from build123d import *

# Parameters (mm, degrees)
EXTRUDE_1_DEPTH     = 5
SKETCH_4_W          = 22
SKETCH_4_H          = 15
SKETCH_4_W_2        = 15
SKETCH_4_H_2        = 22
EXTRUDE_3_DEPTH     = 40
CUT_EXTRUDE_1_REACH = 93.549
CUT_EXTRUDE_2_REACH = 93.549
CUT_EXTRUDE_3_REACH = 93.549
CUT_EXTRUDE_4_REACH = 93.549


with BuildPart() as part:
    # 草图1 → 凸台-拉伸1 (new body)
    with BuildSketch(Plane(origin=(0, 0, 0), x_dir=(1, 0, 0), z_dir=(0, 1, 0))):
        with BuildLine():
            ThreePointArc((29.047375097, 7.5), (21.213203436, 21.213203436), (7.5, 29.047375097))
            Line((7.5, 29.047375097), (7.5, 18.540496218))
            ThreePointArc((7.5, 18.540496218), (14.142135624, 14.142135624), (18.540496218, 7.5))
            Line((18.540496218, 7.5), (29.047375097, 7.5))
        make_face()
        with BuildLine():
            ThreePointArc((30, 0), (29.760890888, 3.780128774), (29.047375097, 7.5))
            Line((29.047375097, 7.5), (18.540496218, 7.5))
            ThreePointArc((18.540496218, 7.5), (19.63173355, 3.820345249), (20, 0))
            ThreePointArc((20, 0), (19.63173355, -3.820345249), (18.540496218, -7.5))
            Line((18.540496218, -7.5), (29.047375097, -7.5))
            ThreePointArc((29.047375097, -7.5), (29.760890888, -3.780128774), (30, 0))
        make_face()
        with BuildLine():
            Line((52.5, 7.5), (29.047375097, 7.5))
            ThreePointArc((29.047375097, 7.5), (29.760890888, 3.780128774), (30, 0))
            ThreePointArc((30, 0), (29.760890888, -3.780128774), (29.047375097, -7.5))
            Line((29.047375097, -7.5), (52.5, -7.5))
            Line((52.5, -7.5), (52.5, 7.5))
        make_face()
        with BuildLine():
            ThreePointArc((7.5, -29.047375097), (21.213203436, -21.213203436), (29.047375097, -7.5))
            Line((29.047375097, -7.5), (18.540496218, -7.5))
            ThreePointArc((18.540496218, -7.5), (14.142135624, -14.142135624), (7.5, -18.540496218))
            Line((7.5, -18.540496218), (7.5, -29.047375097))
        make_face()
        with BuildLine():
            ThreePointArc((7.5, -29.047375097), (0, -30), (-7.5, -29.047375097))
            Line((-7.5, -29.047375097), (-7.5, -52.5))
            Line((-7.5, -52.5), (7.5, -52.5))
            Line((7.5, -52.5), (7.5, -29.047375097))
        make_face()
        with BuildLine():
            Line((-7.5, -18.540496218), (-7.5, -29.047375097))
            ThreePointArc((-7.5, -29.047375097), (0, -30), (7.5, -29.047375097))
            Line((7.5, -29.047375097), (7.5, -18.540496218))
            ThreePointArc((7.5, -18.540496218), (0, -20), (-7.5, -18.540496218))
        make_face()
        with BuildLine():
            Line((-18.540496218, -7.5), (-29.047375097, -7.5))
            ThreePointArc((-29.047375097, -7.5), (-21.213203436, -21.213203436), (-7.5, -29.047375097))
            Line((-7.5, -29.047375097), (-7.5, -18.540496218))
            ThreePointArc((-7.5, -18.540496218), (-14.142135624, -14.142135624), (-18.540496218, -7.5))
        make_face()
        with BuildLine():
            Line((-18.540496218, 7.5), (-29.047375097, 7.5))
            ThreePointArc((-29.047375097, 7.5), (-30, 0), (-29.047375097, -7.5))
            Line((-29.047375097, -7.5), (-18.540496218, -7.5))
            ThreePointArc((-18.540496218, -7.5), (-20, 0), (-18.540496218, 7.5))
        make_face()
        with BuildLine():
            ThreePointArc((-29.047375097, -7.5), (-30, 0), (-29.047375097, 7.5))
            Line((-29.047375097, 7.5), (-52.5, 7.5))
            Line((-52.5, 7.5), (-52.5, -7.5))
            Line((-52.5, -7.5), (-29.047375097, -7.5))
        make_face()
        with BuildLine():
            Line((-7.5, 18.540496218), (-7.5, 29.047375097))
            ThreePointArc((-7.5, 29.047375097), (-21.213203436, 21.213203436), (-29.047375097, 7.5))
            Line((-29.047375097, 7.5), (-18.540496218, 7.5))
            ThreePointArc((-18.540496218, 7.5), (-14.142135624, 14.142135624), (-7.5, 18.540496218))
        make_face()
        with BuildLine():
            ThreePointArc((7.5, 29.047375097), (0, 30), (-7.5, 29.047375097))
            Line((-7.5, 29.047375097), (-7.5, 18.540496218))
            ThreePointArc((-7.5, 18.540496218), (0, 20), (7.5, 18.540496218))
            Line((7.5, 18.540496218), (7.5, 29.047375097))
        make_face()
        with BuildLine():
            Line((7.5, 52.5), (-7.5, 52.5))
            Line((-7.5, 52.5), (-7.5, 29.047375097))
            ThreePointArc((-7.5, 29.047375097), (0, 30), (7.5, 29.047375097))
            Line((7.5, 29.047375097), (7.5, 52.5))
        make_face()
    extrude(amount=EXTRUDE_1_DEPTH)

    # 草图4 → 凸台-拉伸3 (add)
    with BuildSketch(Plane(origin=(0, 5, 0), x_dir=(1, 0, 0), z_dir=(0, 1, 0))):
        with Locations((-41.5, 0)):
            Rectangle(SKETCH_4_W, SKETCH_4_H)
        with Locations((0, 41.5)):
            Rectangle(SKETCH_4_W_2, SKETCH_4_H_2)
        with Locations((41.5, 0)):
            Rectangle(SKETCH_4_W, SKETCH_4_H)
        with Locations((0, -41.5)):
            Rectangle(SKETCH_4_W_2, SKETCH_4_H_2)
    extrude(amount=EXTRUDE_3_DEPTH)

    # 草图5 → 切除-拉伸1 (cut, up to next)
    with BuildSketch(Plane.XY.offset(7.5), mode=Mode.PRIVATE) as cut_extrude_1_sk1:
        Polygon((-52.5, 22.5), (-30.5, 45), (-52.5, 45), align=None)
    cut_extrude_1_tool1 = extrude(cut_extrude_1_sk1.sketch, amount=-CUT_EXTRUDE_1_REACH, mode=Mode.PRIVATE) & part.part
    # 草图5 → 切除-拉伸1 (cut, up to next)
    with BuildSketch(Plane.XY.offset(7.5), mode=Mode.PRIVATE) as cut_extrude_1_sk2:
        Polygon((-35.5, 5), (-30.5, 5), (-30.5, 25), align=None)
    cut_extrude_1_tool2 = extrude(cut_extrude_1_sk2.sketch, amount=-CUT_EXTRUDE_1_REACH, mode=Mode.PRIVATE) & part.part
    add(cut_extrude_1_tool1.solids().sort_by_distance((-45.166667, 37.5, 7.5))[0], mode=Mode.SUBTRACT)
    add(cut_extrude_1_tool2.solids().sort_by_distance((-32.166667, 11.666667, 7.5))[0], mode=Mode.SUBTRACT)

    # 草图6 → 切除-拉伸2 (cut, up to next)
    with BuildSketch(Plane.ZY.offset(7.5), mode=Mode.PRIVATE) as cut_extrude_2_sk1:
        Polygon((-52.5, 22.5), (-30.5, 45), (-52.5, 45), align=None)
    cut_extrude_2_tool1 = extrude(cut_extrude_2_sk1.sketch, amount=-CUT_EXTRUDE_2_REACH, mode=Mode.PRIVATE) & part.part
    # 草图6 → 切除-拉伸2 (cut, up to next)
    with BuildSketch(Plane.ZY.offset(7.5), mode=Mode.PRIVATE) as cut_extrude_2_sk2:
        Polygon((-35.5, 5), (-30.5, 5), (-30.5, 25), align=None)
    cut_extrude_2_tool2 = extrude(cut_extrude_2_sk2.sketch, amount=-CUT_EXTRUDE_2_REACH, mode=Mode.PRIVATE) & part.part
    add(cut_extrude_2_tool1.solids().sort_by_distance((-7.5, 37.5, -45.166667))[0], mode=Mode.SUBTRACT)
    add(cut_extrude_2_tool2.solids().sort_by_distance((-7.5, 11.666667, -32.166667))[0], mode=Mode.SUBTRACT)

    # 草图7 → 切除-拉伸3 (cut, up to next)
    with BuildSketch(Plane(origin=(0, 0, -7.5), x_dir=(-1, 0, 0), z_dir=(0, 0, -1)), mode=Mode.PRIVATE) as cut_extrude_3_sk1:
        Polygon((-52.5, 22.5), (-30.5, 45), (-52.5, 45), align=None)
    cut_extrude_3_tool1 = extrude(cut_extrude_3_sk1.sketch, amount=-CUT_EXTRUDE_3_REACH, mode=Mode.PRIVATE) & part.part
    # 草图7 → 切除-拉伸3 (cut, up to next)
    with BuildSketch(Plane(origin=(0, 0, -7.5), x_dir=(-1, 0, 0), z_dir=(0, 0, -1)), mode=Mode.PRIVATE) as cut_extrude_3_sk2:
        Polygon((-35.5, 5), (-30.5, 5), (-30.5, 25), align=None)
    cut_extrude_3_tool2 = extrude(cut_extrude_3_sk2.sketch, amount=-CUT_EXTRUDE_3_REACH, mode=Mode.PRIVATE) & part.part
    add(cut_extrude_3_tool1.solids().sort_by_distance((45.166667, 37.5, -7.5))[0], mode=Mode.SUBTRACT)
    add(cut_extrude_3_tool2.solids().sort_by_distance((32.166667, 11.666667, -7.5))[0], mode=Mode.SUBTRACT)

    # 草图8 → 切除-拉伸4 (cut, up to next)
    with BuildSketch(Plane(origin=(7.5, 0, 0), x_dir=(0, 0, -1), z_dir=(1, 0, 0)), mode=Mode.PRIVATE) as cut_extrude_4_sk1:
        Polygon((-52.5, 22.5), (-30.5, 45), (-52.5, 45), align=None)
    cut_extrude_4_tool1 = extrude(cut_extrude_4_sk1.sketch, amount=-CUT_EXTRUDE_4_REACH, mode=Mode.PRIVATE) & part.part
    # 草图8 → 切除-拉伸4 (cut, up to next)
    with BuildSketch(Plane(origin=(7.5, 0, 0), x_dir=(0, 0, -1), z_dir=(1, 0, 0)), mode=Mode.PRIVATE) as cut_extrude_4_sk2:
        Polygon((-35.5, 5), (-30.5, 5), (-30.5, 25), align=None)
    cut_extrude_4_tool2 = extrude(cut_extrude_4_sk2.sketch, amount=-CUT_EXTRUDE_4_REACH, mode=Mode.PRIVATE) & part.part
    add(cut_extrude_4_tool1.solids().sort_by_distance((7.5, 37.5, 45.166667))[0], mode=Mode.SUBTRACT)
    add(cut_extrude_4_tool2.solids().sort_by_distance((7.5, 11.666667, 32.166667))[0], mode=Mode.SUBTRACT)


solid = part.part
For this review, take the finished solid that the model builds, in its own axes (mm). A direction names the side the tool comes from. Round coordinates to 2 decimals unless told otherwise and drop trailing zeros. Loops run counter-clockwise (first coordinate to the right, second up) from the corner with the lowest first, then second, coordinate; pieces in that order, holes last. Notation, with made-up numbers: (30, -32) - (73, -32) arc R26 ccw to (73, 7) - close; hole circle Ø3 at (-35.75, -10.75). An arc over 180 degrees is marked (long way). One line per item, written item: value. Start each with the question number.
Item 1: For faces 1 (the flat face through (0, 15, 33)), 2 (the flat face through (0, 35, 30.5)), 3 (the flat face through (7.5, 17, 41)), list the 3-axis set-ups (+Z, -Z, +X, -X, +Y, -Y) from which the entire face can be reached by the end or side of a thin tool; tool diameter is ignored.
Item 2: Take a section at A-A (y = 9). Give the boundary of the cut face in (x, z), plus the area to 3 significant figures.
Item 3: Take a section at B-B (z = 2). Give the boundary of the cut face in (x, y).
Item 4: Clearance check with flat-ended pins moving along their axes: pin 1 Ø3 at (x, y) = (31.5, 31.5) entering from -Z; pin 2 Ø4 at (x, y) = (-34.5, 26) entering from +Z; pin 3 Ø7.5 at (y, z) = (30, -1.5) entering from -X; pin 4 Ø6 at (y, z) = (10, -31) entering from +X. State where each tip first meets the part, or that it passes through.
Item 5: The part is to be moulded in two halves that separate along Z. For faces 4 (the flat face through (-41, 17, -7.5)), 5 (the flat face through (0, 35, -30.5)), 6 (the flat face through (15, 5, 15)), 7 (the flat face through (-30.5, 35, 0)), say which applies: +Z half, -Z half, draft (parallel to the pull), parting line (faces both ways), or undercut.
Item 6: For L1, parallel to Z at x = -36, y = 37; L2, parallel to X at y = 9, z = -5, list the stretches that pass through material, from the lowest coordinate up.
Item 7: Take a section at C-C (x = -3). Give the boundary of the cut face in (y, z).
Item 8: Take a section at D-D (z = -11.5). Give the boundary of the cut face in (x, y).
Answer below:
1. face 1: +X, -X
1. face 2: +X, -X, +Y
1. face 3: +Z, +X, +Y, -Y
2. outline: (-52.5, -7.5) - (-34.5, -7.5) - (-34.5, 7.5) - (-52.5, 7.5) - close; (-7.5, -52.5) - (7.5, -52.5) - (7.5, -34.5) - (-7.5, -34.5) - close; (-7.5, 34.5) - (7.5, 34.5) - (7.5, 52.5) - (-7.5, 52.5) - close; (34.5, -7.5) - (52.5, -7.5) - (52.5, 7.5) - (34.5, 7.5) - close
2. area: 1,080 mm2
3. outline: (-52.5, 0) - (-19.9, 0) - (-19.9, 5) - (-35.5, 5) - (-30.5, 25) - (-30.5, 45) - (-52.5, 22.5) - close; (19.9, 0) - (52.5, 0) - (52.5, 22.5) - (30.5, 45) - (30.5, 25) - (35.5, 5) - (19.9, 5) - close
4. pin 1: stops at z = -7.5
4. pin 2: stops at z = 7.5
4. pin 3: stops at x = -48.83
4. pin 4: passes through
5. face 4: -Z half
5. face 5: undercut
5. face 6: undercut
5. face 7: draft
6. L1: z = -7.5 to 7.5
6. L2: x = -52.5 to -34.5, 34.5 to 52.5
7. outline: (0, -52.5) - (22.5, -52.5) - (45, -30.5) - (25, -30.5) - (5, -35.5) - (5, -19.77) - (0, -19.77) - close; (0, 19.77) - (5, 19.77) - (5, 35.5) - (25, 30.5) - (45, 30.5) - (22.5, 52.5) - (0, 52.5) - close
8. outline: (-27.71, 0) - (-16.36, 0) - (-16.36, 5) - (-27.71, 5) - close; (16.36, 0) - (27.71, 0) - (27.71, 5) - (16.36, 5) - close
